Input: part model. Units: mm. Frame: model coordinates. Round coordinates to 2 decimals unless told otherwise and drop trailing zeros. Loops run counter-clockwise (first coordinate to the right, second up) from the corner with the lowest first, then second, coordinate; pieces in that order, holes last. Notation, with made-up numbers: M -24.5,44.5 L 0.5,44.5 A12 cw 0.5,66.5 Z; hole C 25,24.5 d6. An arc over 180 degrees is marked long. Put each result on its own line as item: value. Start each with the question number.
1) Section B-B on y = -3.1. State how many separate pieces and enclosed holes the cut face has, plus the area to 3 significant figures.
2) Pin query (flat end, axial travel): pin 1 (2.5 mm diameter, centred on x = -19, y = -2.5, fed in from +Z); pin 2 (2.5 mm diameter, centred on y = -2, z = 80.5, fed in from -X); pin 3 (1.5 mm diameter, centred on y = -2, z = 79.5, fed in from -X). Return the tip coordinate at first contact, or that it passes through.
3) Section D-D on x = 32.5. Output: boundary loops of the cut face in (y, z), plus the area to 3 significant figures.
4) Section A-A on z = 24.5. Output: boundary loops of the cut face in (x, y), plus the area to 3 significant figures.
5) Section C-C on z = 79.5. Output: boundary loops of the cut face in (x, y).
6) Line query: probe 1 along X at (y, z) = (-2.3, 67); probe 2 along Z at (x, y) = (36, -3.85); probe 3 along X at (y, z) = (-3, 77). Output: solid intervals per line, ascending.
from build123d import *

# Parameters (mm, degrees)
F0_W     = 6
F0_H     = 6
F0_W_2   = 1.507329056
F0_H_2   = 5.8719553053
F0_W_3   = 8.6
F0_H_3   = 8.6
F1_DEPTH = 5


with BuildPart() as f1:
    # F0 (on Front) → F1 (new body)
    with BuildSketch(Plane.XZ):
        Polygon((-40, 10), (-40, 0), (-1.507329056, 0), (-1.507329056, 5.8719553053), (0, 5.8719553053), (0, 70), (-40, 70), (-40, 60), (-35, 60), (-35, 50), (-40, 50), (-40, 40), (-35, 40), (-35, 30), (-40, 30), (-40, 20), (-35, 20), (-35, 10), align=None)
        with Locations((-20, 15)):
            Rectangle(F0_W, F0_H, mode=Mode.SUBTRACT)
        with Locations((-20, 25)):
            Rectangle(F0_W, F0_H, mode=Mode.SUBTRACT)
        with Locations((-20, 35)):
            Rectangle(F0_W, F0_H, mode=Mode.SUBTRACT)
        with Locations((-20, 45)):
            Rectangle(F0_W, F0_H, mode=Mode.SUBTRACT)
        with Locations((-20, 55)):
            Rectangle(F0_W, F0_H, mode=Mode.SUBTRACT)
        with Locations((-20, 65)):
            Rectangle(F0_W, F0_H, mode=Mode.SUBTRACT)
        with Locations((-0.753664528, 2.9359776527)):
            Rectangle(F0_W_2, F0_H_2)
        with Locations((0.753664528, 2.9359776527)):
            Rectangle(F0_W_2, F0_H_2)
        Polygon((0, 70), (0, 5.8719553053), (1.507329056, 5.8719553053), (1.507329056, 0), (40, 0), (40, 10), (35, 10), (35, 20), (40, 20), (40, 30), (35, 30), (35, 40), (40, 40), (40, 50), (35, 50), (35, 60), (40, 60), (40, 70), align=None)
        with Locations((20, 15)):
            Rectangle(F0_W, F0_H, mode=Mode.SUBTRACT)
        with Locations((20, 25)):
            Rectangle(F0_W, F0_H, mode=Mode.SUBTRACT)
        with Locations((20, 35)):
            Rectangle(F0_W, F0_H, mode=Mode.SUBTRACT)
        with Locations((20, 45)):
            Rectangle(F0_W, F0_H, mode=Mode.SUBTRACT)
        with Locations((20, 55)):
            Rectangle(F0_W, F0_H, mode=Mode.SUBTRACT)
        with Locations((20, 65)):
            Rectangle(F0_W, F0_H, mode=Mode.SUBTRACT)
        Polygon((-40, 70), (0, 70), (40, 70), (14.1260570447, 94.4179981875), (0, 107.7491721764), (-14.1260570447, 94.4179981875), align=None)
        with Locations((-15.7, 79.6245860882)):
            Rectangle(F0_W_3, F0_H_3, mode=Mode.SUBTRACT)
        with Locations((15.7, 79.6245860882)):
            Rectangle(F0_W_3, F0_H_3, mode=Mode.SUBTRACT)
        with BuildLine():
            ThreePointArc((0, 101.3324183106), (3.7476659403, 99.7800842509), (5.3, 96.0324183106))
            ThreePointArc((5.3, 96.0324183106), (3.7476659403, 92.2847523704), (0, 90.7324183106))
            ThreePointArc((0, 90.7324183106), (-3.7476659403, 92.2847523704), (-5.3, 96.0324183106))
            ThreePointArc((-5.3, 96.0324183106), (-3.7476659403, 99.7800842509), (0, 101.3324183106))
        make_face(mode=Mode.SUBTRACT)
    extrude(amount=F1_DEPTH)


solid = f1.part
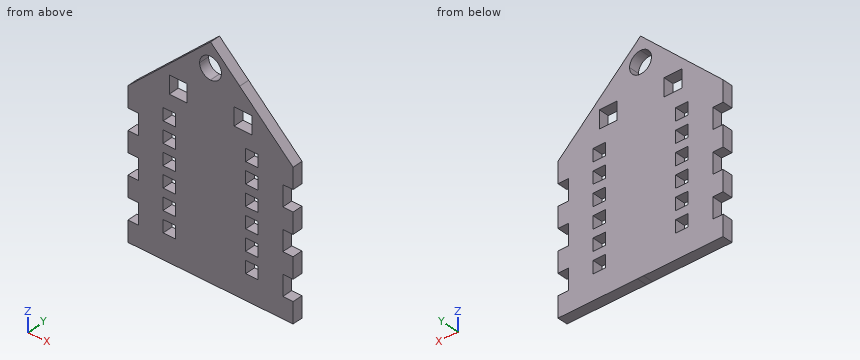
Geometry results:
1. separate pieces: 1
1. enclosed holes: 15
1. area: 6,140 mm²
2. pin 1: stops at z = 91
2. pin 2: stops at x = -30.2
2. pin 3: stops at x = -30.73
3. outline: M -5,0 L 0,0 L 0,77.08 L -5,77.08 Z
3. area: 385 mm²
4. outline: M -40,-5 L -23,-5 L -23,0 L -40,0 Z; M -17,-5 L 17,-5 L 17,0 L -17,0 Z; M 23,-5 L 40,-5 L 40,0 L 23,0 Z
4. area: 340 mm²
5. outline: M -29.93,-5 L -20,-5 L -20,0 L -29.93,0 Z; M -11.4,-5 L 11.4,-5 L 11.4,0 L -11.4,0 Z; M 20,-5 L 29.93,-5 L 29.93,0 L 20,0 Z
6. probe 1: x = -40 to -23, -17 to 17, 23 to 40
6. probe 2: z = 0 to 10, 20 to 30, 40 to 50, 60 to 73.77
6. probe 3: x = -32.58 to -20, -11.4 to 11.4, 20 to 32.58
